Check sheet for the modelled part. Datum: model origin and axes. Units: mm. A direction names the side the tool comes from. Round coordinates to 2 decimals unless told otherwise and drop trailing zeros. Loops run counter-clockwise (first coordinate to the right, second up) from the corner with the lowest first, then second, coordinate; pieces in that order, holes last. Notation, with made-up numbers: (30, 26.5) -> (55, 26.5) arc R31 ccw to (55, 56.5) -> close; hole circle Ø7 at (-13.5, -24.75). An arc over 180 degrees is marked (long way). One line per question, with ' | ' between items.
```python
from build123d import *

# Parameters (mm, degrees)
SKETCH1_R             = 1.9812
SKETCH1_R_2           = 3.175
BOSS_EXTRUDE1_DEPTH   = 15.621
FILLET1_R             = 5.08
FILLET2_R             = 1.905
SKETCH2_R             = 11.25
CUT_EXTRUDE1_DEPTH    = 8.769999986
BOSS_EXTRUDE2_START   = 1.27
SKETCH3_R             = 5.715
SKETCH3_R_2           = 1.9812
BOSS_EXTRUDE2_DEPTH   = 1.27
FILLET3_R             = 1.27
BODY_MOVE_COPY1_ANGLE = 180
SKETCH4_W             = 19.05
SKETCH4_H             = 1.778
CUT_EXTRUDE2_DEPTH    = 67.693165799
FILLET4_R             = 1.27
FILLET5_R             = 12.7
CUT_EXTRUDE3_DEPTH    = 3.175
SKETCH6_R             = 1.27
CUT_EXTRUDE4_DEPTH    = 67.693165799
FILLET6_R             = 3.81
FILLET7_R             = 2.032
SKETCH7_R             = 2.54
CUT_EXTRUDE5_DEPTH    = 8.89


with BuildPart() as part:
    # Sketch1 → Boss-Extrude1 (new body)
    with BuildSketch(Plane.XY):
        with BuildLine():
            Line((-9.525, 0), (-9.525, 28.2))
            Line((-9.525, 28.2), (53.5118, 28.2))
            Line((53.5118, 28.2), (53.5118, 23.4375))
            Line((53.5118, 23.4375), (36.0493, 23.4375))
            Line((36.0493, 23.4375), (9.525, 12.7))
            Line((9.525, 12.7), (9.525, 0))
            ThreePointArc((9.525, 0), (0, -9.525), (-9.525, 0))
        make_face()
        with Locations(Location((0, 0, 0), (0, 0, 180))):
            Circle(SKETCH1_R, mode=Mode.SUBTRACT)
        with Locations(Location((0, 15.5, 0), (0, 0, 180))):
            Circle(SKETCH1_R_2, mode=Mode.SUBTRACT)
    extrude(amount=BOSS_EXTRUDE1_DEPTH)

    # Fillet1
    fillet1_edges = [part.edges().sort_by_distance(p)[0] for p in [
        (36.0493, 23.4375, 7.8105),
        (9.525, 12.7, 7.8105),
    ]]
    fillet(fillet1_edges, radius=FILLET1_R)

    # Fillet2
    fillet2_edges = [part.edges().sort_by_distance(p)[0] for p in [
        (53.5118, 28.2, 7.8105),
        (53.5118, 23.4375, 7.8105),
    ]]
    fillet(fillet2_edges, radius=FILLET2_R)

    # Sketch2 → Cut-Extrude1 (cut)
    with BuildSketch(Plane(origin=(0, 0, 0), x_dir=(-1, 0, 0), z_dir=(0, 0, -1))):
        Circle(SKETCH2_R)
    extrude(amount=-CUT_EXTRUDE1_DEPTH, mode=Mode.SUBTRACT)

    # Sketch3 → Boss-Extrude2 (add)
    with BuildSketch(Plane(origin=(0, 0, 8.769999986), x_dir=(-1, 0, 0), z_dir=(0, 0, -1)).offset(BOSS_EXTRUDE2_START)):
        Circle(SKETCH3_R)
        Circle(SKETCH3_R_2, mode=Mode.SUBTRACT)
    extrude(amount=-BOSS_EXTRUDE2_DEPTH)

    # Fillet3
    # the kernel refuses this fillet: 1.27 mm, written as the material it takes off along each edge
    with BuildSketch(Plane(origin=(-9.525, 5.986390816, 8.769999986), x_dir=(0, 1, 0), z_dir=(0, 0, -1))) as fillet3_piece_1:
        with BuildLine():
            CenterArc((3.426651997, 1.27), FILLET3_R, 138.750058465, 131.249941535)
            ThreePointArc((2.471814587, 2.107368211), (1.312365255, 0.964003573), (0, 0))
            Line((0, 0), (3.426651997, 0))
        make_face()
    extrude(amount=17.336629979, mode=Mode.SUBTRACT)
    with BuildSketch(Plane(origin=(9.525, 5.986390816, 8.769999986), x_dir=(-0.6487196430292314, 0.761027479627396, 0), z_dir=(0, 0, -1))) as fillet3_piece_2:
        with BuildLine():
            CenterArc((3.429739885, 1.256710275), FILLET3_R, 131.670192506, 130.033722059)
            Line((2.585390755, 2.205380158), (2.500955842, 2.300247146))
            ThreePointArc((2.500955842, 2.300247146), (2.421102629, 2.230690584), (-0.082387395, 0.09665049))
            Line((-0.082387395, 0.09665049), (0.018324651, -0.125671027))
            ThreePointArc((0.018324651, -0.125671027), (1.623246685, -0.009276057), (3.228168719, -0.125671027))
            Line((3.228168719, -0.125671027), (3.24649337, 0))
        make_face()
    extrude(amount=17.26556758, mode=Mode.SUBTRACT)


with BuildPart() as part_1:
    # Body-Move/Copy1: moved
    add(part.part.rotate(Axis((0, 6.7975, 6.35), (1, 0, 0)), BODY_MOVE_COPY1_ANGLE))

    # Sketch4 → Cut-Extrude2 (cut, through all)
    with BuildSketch(Plane.XZ.offset(14.605)):
        with Locations((43.9868, 11.811)):
            Rectangle(SKETCH4_W, SKETCH4_H)
    extrude(amount=-CUT_EXTRUDE2_DEPTH, mode=Mode.SUBTRACT)

    # Fillet4
    fillet4_edges = [part_1.edges().sort_by_distance(p)[0] for p in [
        (34.4618, -9.199852268, 11.811),
        (34.4618, -14.605, 11.811),
    ]]
    fillet(fillet4_edges, radius=FILLET4_R)

    # Fillet5
    fillet5_edges = [part_1.edges().sort_by_distance(p)[0] for p in [
        (-9.525, -14.605, 4.8895),
    ]]
    fillet(fillet5_edges, radius=FILLET5_R)

    # Sketch5 → Cut-Extrude3 (cut)
    with BuildSketch(Plane.XY.offset(12.7)):
        with BuildLine():
            ThreePointArc((-5.408855404, 0.750246956), (-5.911348625, -3.072052101), (-3.993935769, -6.416599523))
            ThreePointArc((-3.993935769, -6.416599523), (-15.75834811, -5.016102801), (-5.408855404, 0.750246956))
        make_face()
    extrude(amount=-CUT_EXTRUDE3_DEPTH, mode=Mode.SUBTRACT)

    # Sketch6 → Cut-Extrude4 (cut, through all)
    with BuildSketch(Plane.XZ.offset(14.605)):
        with Locations(Location((11.125, 8.4455, 0), (0, 0, 270))):
            Circle(SKETCH6_R)
        with BuildLine():
            Line((39.416476, 7.8867), (40.686476, 7.8867))
            ThreePointArc((40.686476, 7.8867), (42.667676, 5.9055), (40.686476, 3.9243))
            Line((40.686476, 3.9243), (39.416476, 3.9243))
            ThreePointArc((39.416476, 3.9243), (37.435276, 5.9055), (39.416476, 7.8867))
        make_face()
    extrude(amount=-CUT_EXTRUDE4_DEPTH, mode=Mode.SUBTRACT)

    # Fillet6
    # the kernel refuses this fillet: 3.81 mm, written as the material it adds along each edge
    with BuildSketch(Plane(origin=(-5.408855404, 0.750246956, 12.7), x_dir=(-0.2519962053537531, -0.9677282224298872, 0), z_dir=(0, 0, -1))) as fillet6_piece_1:
        with BuildLine():
            CenterArc((3.176013598, 3.732834284), FILLET6_R, 169.868712544, 88.580194717)
            Line((-0.574578104, 4.403029693), (-0.649589938, 4.416433601))
            ThreePointArc((-0.649589938, 4.416433601), (-0.768643464, 2.138699984), (-0.067078157, -0.036151913))
            Line((-0.067078157, -0.036151913), (0.015258417, -0.074656686))
            ThreePointArc((0.015258417, -0.074656686), (1.20654638, 0.045836272), (2.397834343, -0.074656686))
            Line((2.397834343, -0.074656686), (2.41309276, 0))
        make_face()
    extrude(amount=14.275903813)
    with BuildSketch(Plane(origin=(-3.993935769, -6.416599523, 12.7), x_dir=(-0.7064973640588543, -0.7077156735426245, 0), z_dir=(0, 0, -1))) as fillet6_piece_2_section:
        with BuildLine():
            CenterArc((3.250231885, 3.662124285), FILLET6_R, 199.612026349, 86.403394204)
            Line((-0.338738664, 2.383300453), (-0.410518075, 2.357723976))
            ThreePointArc((-0.410518075, 2.357723976), (-0.12457926, 1.198016243), (-0.076063221, 0.004563593))
            Line((-0.076063221, 0.004563593), (-0.026317873, -0.071510905))
            ThreePointArc((-0.026317873, -0.071510905), (2.150697936, -0.459393071), (4.322419151, -0.073242486))
            Line((4.322419151, -0.073242486), (4.301395871, 0))
        make_face()
    fillet6_piece_2 = extrude(amount=13.928489678, mode=Mode.PRIVATE)
    fillet6_piece_2 = fillet6_piece_2 & Plane(origin=(3.175, -1.905, 11.1125), x_dir=(-1, 0, 0), z_dir=(0, 0, -1)) * Cylinder(12.7, 46, mode=Mode.PRIVATE)
    add(fillet6_piece_2)

    # Fillet7
    fillet7_edges = [part_1.edges().sort_by_distance(p)[0] for p in [
        (-5.910770655, -3.074975831, 9.525),
        (-5.253622107, -7.292001089, 9.525),
        (-6.956861839, 1.129272671, 9.525),
    ]]
    fillet(fillet7_edges, radius=FILLET7_R)

    # Sketch7 → Cut-Extrude5 (cut)
    with BuildSketch(Plane.XZ.offset(14.605)):
        with Locations(Location((11.125, 8.4455, 0), (0, 0, 270))):
            Circle(SKETCH7_R)
    extrude(amount=-CUT_EXTRUDE5_DEPTH, mode=Mode.SUBTRACT)


solid = part_1.part
```
(1) Set-up check for faces 4 (the face through (-2.5, 13.5, 5.2)), 5 (the face through (34.462, -12, 12)), 6 (the face through (-6.984, 1.16, 12.137)), 7 (the face through (-8.761, 5.347, 8.254)), 8 (the face through (-2, 8, 3.93)): record each of +Z, -Z, +X, -X, +Y, -Y from which the full face is reachable in a straight line by a thin tool's end or side.
Answer:
face 4: +Z, +X, -X, +Y | face 5: +Z, +X, +Y, -Y | face 6: +Z, -X | face 7: +Z, +Y | face 8: +Z
(2) Sectioned sample at B-B, the plane y = 17. Record the cut outline in (x, z), and give its area (3 significant figures).
Answer:
outline: (-8.9, -2.92) -> (8.9, -2.92) -> (8.9, 3.93) -> (4.59, 3.93) -> (4.59, 5.2) -> (-4.59, 5.2) -> (-4.59, 3.93) -> (-8.9, 3.93) -> close | area: 134 mm2
(3) Mould release check, pull along Z, two halves, no side actions. Record for faces 1 (the face through (-5.24, -7.25, 12.14)), 2 (the face through (8, 0, -2.921)), 3 (the face through (40, -12, 3.924)): +Z half, -Z half, draft (parallel to the pull), parting line (faces both ways), or undercut.
Answer:
face 1: draft | face 2: -Z half | face 3: undercut
(4) Sectioned sample at A-A, the plane x = 0. Record the cut outline in (y, z) (3 decimals).
Answer:
outline: (-14.202, -2.921) -> (-5.08, -2.921) -> (-5.08, 12.7) -> (-14.202, 12.7) -> close; (1.27, -2.921) -> (11.614, -2.921) -> (11.614, 5.2) -> (7.88, 5.2) -> (7.88, 3.93) -> (2.345, 3.93) -> (2.345, 12.7) -> (1.27, 12.7) -> close; (15.576, -2.921) -> (23.12, -2.921) -> (23.12, 3.93) -> (19.31, 3.93) -> (19.31, 5.2) -> (15.576, 5.2) -> close
(5) Go/stop test with flat-tipped pins: pin 1 (3.5 mm diameter, centred on y = 9, z = 1, fed in from +X) (3 decimals); pin 2 (6 mm diameter, centred on y = -3.5, z = 8, fed in from +X); pin 3 (4 mm diameter, centred on y = 4, z = 8.5, fed in from +X). Record where each tip stops, or that it passes through.
Answer:
pin 1: stops at x = 9.525 | pin 2: stops at x = 27.79 | pin 3: stops at x = 10.04
(6) Sectioned sample at D-D, the plane x = 22. Record the cut outline in (y, z) (3 decimals), and give its area (3 significant figures).
Answer:
outline: (-14.605, -2.921) -> (-4.155, -2.921) -> (-4.155, 12.7) -> (-14.605, 12.7) -> close | area: 163 mm2
(7) Sectioned sample at C-C, the plane x = 31.5. Record the cut outline in (y, z) (3 decimals), and give its area (3 significant figures).
Answer:
outline: (-14.605, -2.921) -> (-8.001, -2.921) -> (-8.001, 12.7) -> (-14.605, 12.7) -> close | area: 103 mm2
(8) Scan lines: probe 1 along Y at (x, z) = (0, 0.75); probe 2 along Y at (x, z) = (48, 8.5) (1 decimal); probe 3 along Z at (x, y) = (-3.5, 8.5). Record each from-to range of solid material in increasing order.
Answer:
probe 1: y = -14.2 to -5.08, 1.27 to 11.61, 15.58 to 23.12 | probe 2: y = -14.6 to -9.8 | probe 3: z = -2.92 to 3.93
